Part model, mm, in its own coordinate system. Face numbers are marked on the shaded views. A direction names the side the tool comes from. Give positions to 0.01 mm unless a question says otherwise; leave off trailing zeros. Order: outer loops, then holes, each group sorted by start corner. A loop starts at its lowest first (then second) coordinate and runs counter-clockwise, first axis right, second up.
1. Probe line 1 (Y direction, x = 5.25, z = 27); line 2 (X direction, y = 4.5, z = 27). List the from-to ranges inside material, lowest first.
2. Which spindle directions (+Z, -Z, +X, -X, +Y, -Y) get a long thin tool onto all of the face, cutting with end or side? Do the marked faces 4, 5 and 6. Say none if no direction does.
3. Drop flat-ended pins along their axis: pin 1 Ø10 at (y, z) = (46.5, 9.5) entering from -X; pin 2 Ø5 at (y, z) = (18.5, 19) entering from +X. Give the stop position or say it passes through.
4. Slice it at A-A on y = 64. List the corners of the cut face in (x, z).
5. Slice it at B-B on x = 22.75. List the corners of the cut face in (y, z), and give its area (3 significant figures).
6. Slice it at D-D on z = 2.25. List the corners of the cut face in (x, y).
7. Mould opens along Y. For the marked faces 1, 2 and 3 say: +Y half, -Y half, draft (parallel to the pull), parting line (faces both ways), or undercut.
8. Slice it at C-C on z = 16.25. List the corners of the cut face in (x, y).
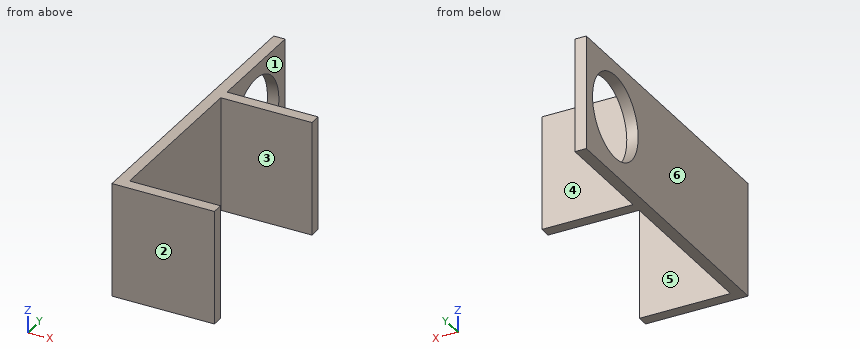
from build123d import *

# Parameters (mm, degrees)
EXTRUDE_1_DEPTH     = 30
SKETCH_2_W          = 3
SKETCH_2_H          = 30
EXTRUDE_2_DEPTH     = 28
CUT_EXTRUDE_1_REACH = 89.824
SKETCH_3_R          = 11


with BuildPart() as part:
    # 草图1 → 凸台-拉伸1 (new body)
    with BuildSketch(Plane.XY):
        Polygon((27, 47), (27, 50), (0, 50), (0, 0), (27, 0), (27, 3), (3, 3), (3, 47), align=None)
    extrude(amount=EXTRUDE_1_DEPTH)

    # 草图2 → 凸台-拉伸2 (add)
    with BuildSketch(Plane(origin=(0, 50, 0), x_dir=(1, 0, 0), z_dir=(0, 1, 0))):
        with Locations((1.5, -15)):
            Rectangle(SKETCH_2_W, SKETCH_2_H)
    extrude(amount=EXTRUDE_2_DEPTH)

    # 草图3 → 切除-拉伸1 (cut, up to next)
    with BuildSketch(Plane.ZY, mode=Mode.PRIVATE) as cut_extrude_1_sk1:
        with Locations((15.518002159, 64)):
            Circle(SKETCH_3_R)
    cut_extrude_1_tool1 = extrude(cut_extrude_1_sk1.sketch, amount=-CUT_EXTRUDE_1_REACH, mode=Mode.PRIVATE) & part.part
    add(cut_extrude_1_tool1.solids().sort_by_distance((0, 64, 15.518002))[0], mode=Mode.SUBTRACT)


solid = part.part
Data:
1. line 1: y = 0 to 3, 47 to 50
1. line 2: x = 0 to 3
2. face 4: +Z, -Z, +X, +Y
2. face 5: +Z, -Z, +X
2. face 6: +Z, -Z, -X, +Y, -Y
3. pin 1: stops at x = 0
3. pin 2: stops at x = 3
4. outline: (0, 0) - (3, 0) - (3, 4.52) - (0, 4.52) - close; (0, 26.52) - (3, 26.52) - (3, 30) - (0, 30) - close
5. outline: (0, 0) - (3, 0) - (3, 30) - (0, 30) - close; (47, 0) - (50, 0) - (50, 30) - (47, 30) - close
5. area: 180 mm2
6. outline: (0, 0) - (27, 0) - (27, 3) - (3, 3) - (3, 47) - (27, 47) - (27, 50) - (3, 50) - (3, 78) - (0, 78) - close
7. face 1: draft
7. face 2: -Y half
7. face 3: undercut
8. outline: (0, 0) - (27, 0) - (27, 3) - (3, 3) - (3, 47) - (27, 47) - (27, 50) - (3, 50) - (3, 53.02) - (0, 53.02) - close; (0, 74.98) - (3, 74.98) - (3, 78) - (0, 78) - close
